Build history of the part. All positions in model axes, mm. A direction names the side the tool comes from. Coordinates: 2 decimals unless noted, no trailing zeros. Order: outer loops, then holes, each group sorted by start corner. A loop starts at its lowest first (then second) coordinate and runs counter-clockwise, first axis right, second up. Notation, with made-up numbers: (-8, 23) - (39, 23) arc R30 ccw to (39, 55) - close; hole circle Ø4 at (0.25, 71.5). An arc over 180 degrees is marked (long way). Write each question's results on one line, items separated by ' | '.
from build123d import *

# Parameters (mm, degrees)
CUT_EXTRUDE1_START             = -0.2
CUT_EXTRUDE1_DEPTH             = 0.2
CUT_EXTRUDE1_START_2           = -7
CUT_EXTRUDE1_2_DEPTH           = 0.1999999
CUT_EXTRUDE1_START_3           = -6.8000001
CUT_EXTRUDE1_3_DEPTH           = 6.6000001
CUT_EXTRUDE1_START_4           = 9.5
CUT_EXTRUDE1_4_DEPTH           = 6.5
SKETCH2_R                      = 3.95
BOSS_EXTRUDE1_DEPTH            = 2.5
CUT_EXTRUDE2_DEPTH             = 22.300469551
SKETCH4_W                      = 2.45
SKETCH4_H                      = 9.5
M2_5_CLEARANCE_HOLE1_D         = 2.7051
M2_5_CLEARANCE_HOLE1_DEPTH     = 9.5
SKETCH7_W                      = 1.35255
SKETCH7_H                      = 10.6
F_3_7_3_7_DIAMETER_HOLE1_D     = 3.7
F_3_7_3_7_DIAMETER_HOLE1_DEPTH = 15.1


with BuildPart() as part:
    # Cut-Extrude1: read off the stored shape, not the designer's step
    # Cut-Extrude1 outline → Cut-Extrude1 (new body)
    with BuildSketch(Plane.XY.offset(CUT_EXTRUDE1_START)):
        with BuildLine():
            ThreePointArc((8.719864541, -6.868330393), (11.819050527, -4.746581358), (15.5, -4))
            Line((15.5, -4), (15.5, 4))
            ThreePointArc((15.5, 4), (11.819050527, 4.746581358), (8.719864541, 6.868330393))
            ThreePointArc((8.719864541, 6.868330393), (-11.1, 0), (8.719864541, -6.868330393))
        make_face()
    extrude(amount=CUT_EXTRUDE1_DEPTH)



with BuildPart() as body_2:
    # Cut-Extrude1 2 outline → Cut-Extrude1 2 (new body)
    with BuildSketch(Plane.XY.offset(CUT_EXTRUDE1_START_2)):
        with BuildLine():
            ThreePointArc((8.719864541, -6.868330393), (11.819050527, -4.746581358), (15.5, -4))
            Line((15.5, -4), (15.5, 4))
            ThreePointArc((15.5, 4), (11.819050527, 4.746581358), (8.719864541, 6.868330393))
            ThreePointArc((8.719864541, 6.868330393), (-11.1, 0), (8.719864541, -6.868330393))
        make_face()
    extrude(amount=CUT_EXTRUDE1_2_DEPTH)


with BuildPart() as part_1:
    add(part.part)

    add(body_2.part)  # Cut-Extrude1 3 merges body 2
    # Cut-Extrude1 3 outline → Cut-Extrude1 3 (add)
    with BuildSketch(Plane.XY.offset(CUT_EXTRUDE1_START_3)):
        with BuildLine():
            ThreePointArc((8.719864541, -6.868330393), (11.819050527, -4.746581358), (15.5, -4))
            Line((15.5, -4), (15.5, 4))
            ThreePointArc((15.5, 4), (11.819050527, 4.746581358), (8.719864541, 6.868330393))
            ThreePointArc((8.719864541, 6.868330393), (-11.1, 0), (8.719864541, -6.868330393))
        make_face()
    extrude(amount=CUT_EXTRUDE1_3_DEPTH)

    # Cut-Extrude1 4 outline → Cut-Extrude1 4 (cut)
    with BuildSketch(Plane.YZ.offset(CUT_EXTRUDE1_START_4)):
        with BuildLine():
            ThreePointArc((4, -6.8), (6.016591059, -3.5), (4, -0.2))
            Line((4, -0.2), (4, -6.8))
        make_face()
    extrude(amount=CUT_EXTRUDE1_4_DEPTH, mode=Mode.SUBTRACT)

    # Sketch2 → Boss-Extrude1 (add)
    with BuildSketch(Plane.XY):
        Circle(SKETCH2_R)
    extrude(amount=BOSS_EXTRUDE1_DEPTH)

    # Sketch3 → Cut-Extrude2 (cut, through all)
    with BuildSketch(Plane(origin=(0, 0, -7), x_dir=(-1, 0, 0), z_dir=(0, 0, -1))):
        with BuildLine():
            Line((-15.5, 0.5), (-15.5, -0.5))
            Line((-15.5, -0.5), (-2.398436991, -0.5))
            ThreePointArc((-2.398436991, -0.5), (-2.45, 0), (-2.398436991, 0.5))
            Line((-2.398436991, 0.5), (-15.5, 0.5))
        make_face()
    extrude(amount=-CUT_EXTRUDE2_DEPTH, mode=Mode.SUBTRACT)

    # Sketch4 → Cut-Revolve1 (revolve, cut)
    with BuildSketch(Plane.XZ):
        with Locations((1.225, -2.25)):
            Rectangle(SKETCH4_W, SKETCH4_H)
    revolve(axis=Axis((0, 0, 2.5), (0, 0, -1)), mode=Mode.SUBTRACT)

    # M2.5 Clearance Hole1
    with Locations(Plane(origin=(0, 0, -7), x_dir=(-1, 0, 0), z_dir=(0, 0, -1))):
        with Locations((5.656516225, 5.657192254), (-5.657192254, 5.656516225), (-5.656516225, -5.657192254), (5.657192254, -5.656516225)):
            Hole(M2_5_CLEARANCE_HOLE1_D / 2, depth=M2_5_CLEARANCE_HOLE1_DEPTH)

    # Sketch7 → M2.5 Clearance Hole2 (revolve, cut)
    with BuildSketch(Plane(origin=(13, -0.5, -3.5), x_dir=(0, 0, 1), z_dir=(1, 0, 0))):
        with Locations((0.676275, 5.3)):
            Rectangle(SKETCH7_W, SKETCH7_H)
    revolve(axis=Axis((13, 5.85, -3.5), (0, -1, 0)), mode=Mode.SUBTRACT)

    # Ø3.7 (3.7) Diameter Hole1
    with Locations(Plane(origin=(0, 4, 0), x_dir=(1, 0, 0), z_dir=(0, 1, 0))):
        with Locations((13, 3.5)):
            Hole(F_3_7_3_7_DIAMETER_HOLE1_D / 2, depth=F_3_7_3_7_DIAMETER_HOLE1_DEPTH)


solid = part_1.part
1. Probe line 1 (Y direction, x = 0, z = -1); line 2 (Y direction, x = -6.5, z = -5.5); line 3 (Z direction, x = -5.5, y = 1.75). List the from-to ranges inside material, lowest first.
Solved:
line 1: y = -11.1 to -2.45, 2.45 to 11.1 | line 2: y = -9 to -6.71, -4.6 to 4.6, 6.71 to 9 | line 3: z = -7 to 0
2. Band-saw the part on C-C on y = 1.5. Give the cut face in (x, z).
Solved:
outline: (-11, -7) - (-1.94, -7) - (-1.94, 2.5) - (-3.65, 2.5) - (-3.65, 0) - (-11, 0) - close; (1.94, -7) - (15.5, -7) - (15.5, 0) - (3.65, 0) - (3.65, 2.5) - (1.94, 2.5) - close; hole circle Ø3.7 at (13, -3.5)
3. Band-saw the part on A-A on z = -3.5. Give the cut face in (x, y).
Solved:
outline: (2.4, -0.5) arc R2.45 cw (long way) to (2.4, 0.5) - (11.15, 0.5) - (11.15, 4) - (9.5, 4) - (9.5, 6.02) - (9.67, 6.02) arc R9.45 cw to (8.72, 6.87) arc R11.1 ccw (long way) to (8.72, -6.87) arc R9.45 cw to (11.15, -5.06) - (11.15, -0.5) - close; (14.85, -4.02) arc R9.45 cw to (15.5, -4) - (15.5, -0.5) - (14.85, -0.5) - close; (14.85, 0.5) - (15.5, 0.5) - (15.5, 4) - (14.85, 4) - close; hole circle Ø2.71 at (-5.66, -5.66); hole circle Ø2.71 at (-5.66, 5.66); hole circle Ø2.71 at (5.66, -5.66); hole circle Ø2.71 at (5.66, 5.66)
4. Drop flat-ended pins along their axis: pin 1 Ø1.5 at (x, z) = (-0.5, 1) entering from +Y; pin 2 Ø6 at (x, y) = (7, -1) entering from +Z; pin 3 Ø6.5 at (x, y) = (0, 0) entering from -Z; pin 4 Ø3 at (x, z) = (11.5, 0) entering from -Y. Give the stop position or say it passes through.
Solved:
pin 1: stops at y = 3.95 | pin 2: stops at z = 0 | pin 3: stops at z = -7 | pin 4: stops at y = -5.77
5. Band-saw the part on B-B on x = 0. Give the cut face in (y, z), then the cut area to 3 significant figures.
Solved:
outline: (-11.1, -7) - (-2.45, -7) - (-2.45, 2.5) - (-3.95, 2.5) - (-3.95, 0) - (-11.1, 0) - close; (2.45, -7) - (11.1, -7) - (11.1, 0) - (3.95, 0) - (3.95, 2.5) - (2.45, 2.5) - close | area: 129 mm2
6. Band-saw the part on D-D on x = 11.5. Give the cut face in (y, z).
Solved:
outline: (-4.89, -7) - (-0.5, -7) - (-0.5, -4.58) - (-4.89, -4.58) - close; (-4.89, -2.42) - (-0.5, -2.42) - (-0.5, 0) - (-4.89, 0) - close; (0.5, -7) - (4.89, -7) - (4.89, -6.16) arc R3.71 cw to (4, -6.8) - (4, -4.58) - (0.5, -4.58) - close; (0.5, -2.42) - (4, -2.42) - (4, -0.2) arc R3.71 cw to (4.89, -0.84) - (4.89, 0) - (0.5, 0) - close
7. Two-plate mould, pull along X, no slides. Class faces 6 (the face through (9.45, 6.19, -3.52)), 7 (the face through (-2.448, -0.101, -2.183)), 8 (the face through (9, 0.5, -3)): +X half, -X half, draft (parallel to the pull), parting line (faces both ways), or undercut.
Solved:
face 6: +X half | face 7: undercut | face 8: draft
8. Tool access for faces 1 (the face through (11.014, -5.133, -3.549)), 2 (the face through (-6.653, 6.571, -3.451)), 3 (the face through (2, -5, 0)), 4 (the face through (11, 4, -3)), 5 (the face through (9, -0.5, -3)): list every direction of +Z, -Z, +X, -X, +Y, -Y with a clear straight run to the whole face (end or side of a thin tool).
Solved:
face 1: +Z, -Z, +X, -Y | face 2: +Z, -Z | face 3: +Z | face 4: +X | face 5: +Z, -Z, +X
